Part model, mm, in its own coordinate system. A direction names the side the tool comes from. Give positions to 0.01 mm unless a question says otherwise; leave off trailing zeros. Write each loop counter-clockwise with the first axis right and the second up, starting at its lowest first coordinate (ties: lowest second). Pieces come first, ordered by that corner, then holes. Notation, with made-up numbers: M -36,-34.75 L 8,-34.75 A18 ccw 8,-11.75 Z; hole C -27.5,89.5 d10. An arc over 180 degrees is marked long. Write item = value, one per line. Start each with the question number.
from build123d import *

# Parameters (mm, degrees)
BOSS_EXTRUDE1_DEPTH = 127
CUT_EXTRUDE1_REACH  = 147.912
SKETCH2_R           = 6
SKETCH2_R_2         = 3.175
CUT_EXTRUDE2_REACH  = 147.912
SKETCH3_R           = 2.75
SKETCH3_W           = 29.8
SKETCH3_H           = 64.8
FILLET1_R           = 2


with BuildPart() as part:
    # Sketch1 → Boss-Extrude1 (new body)
    with BuildSketch(Plane(origin=(0, 0, 0), x_dir=(1, 0, 0), z_dir=(0, 1, 0))):
        Polygon((0, 50.8), (0, 0), (50.8, 0), (50.8, -3.175), (-3.175, -3.175), (-3.175, 50.8), align=None)
    extrude(amount=BOSS_EXTRUDE1_DEPTH)

    # Sketch2 → Cut-Extrude1 (cut, up to next)
    with BuildSketch(Plane(origin=(0, 0, 0), x_dir=(-1, 0, 0), z_dir=(0, 0, -1)), mode=Mode.PRIVATE) as cut_extrude1_sk1:
        with Locations((-25.4, 63.5)):
            Circle(SKETCH2_R)
    cut_extrude1_tool1 = extrude(cut_extrude1_sk1.sketch, amount=-CUT_EXTRUDE1_REACH, mode=Mode.PRIVATE) & part.part
    # Sketch2 → Cut-Extrude1 (cut, up to next)
    with BuildSketch(Plane(origin=(0, 0, 0), x_dir=(-1, 0, 0), z_dir=(0, 0, -1)), mode=Mode.PRIVATE) as cut_extrude1_sk2:
        with Locations((-25.4, 75.5)):
            Circle(SKETCH2_R_2)
    cut_extrude1_tool2 = extrude(cut_extrude1_sk2.sketch, amount=-CUT_EXTRUDE1_REACH, mode=Mode.PRIVATE) & part.part
    # Sketch2 → Cut-Extrude1 (cut, up to next)
    with BuildSketch(Plane(origin=(0, 0, 0), x_dir=(-1, 0, 0), z_dir=(0, 0, -1)), mode=Mode.PRIVATE) as cut_extrude1_sk3:
        with Locations((-13.4, 63.5)):
            Circle(SKETCH2_R_2)
    cut_extrude1_tool3 = extrude(cut_extrude1_sk3.sketch, amount=-CUT_EXTRUDE1_REACH, mode=Mode.PRIVATE) & part.part
    # Sketch2 → Cut-Extrude1 (cut, up to next)
    with BuildSketch(Plane(origin=(0, 0, 0), x_dir=(-1, 0, 0), z_dir=(0, 0, -1)), mode=Mode.PRIVATE) as cut_extrude1_sk4:
        with Locations((-25.4, 51.5)):
            Circle(SKETCH2_R_2)
    cut_extrude1_tool4 = extrude(cut_extrude1_sk4.sketch, amount=-CUT_EXTRUDE1_REACH, mode=Mode.PRIVATE) & part.part
    # Sketch2 → Cut-Extrude1 (cut, up to next)
    with BuildSketch(Plane(origin=(0, 0, 0), x_dir=(-1, 0, 0), z_dir=(0, 0, -1)), mode=Mode.PRIVATE) as cut_extrude1_sk5:
        with Locations((-37.4, 63.5)):
            Circle(SKETCH2_R_2)
    cut_extrude1_tool5 = extrude(cut_extrude1_sk5.sketch, amount=-CUT_EXTRUDE1_REACH, mode=Mode.PRIVATE) & part.part
    add(cut_extrude1_tool1.solids().sort_by_distance((25.4, 63.5, 0))[0], mode=Mode.SUBTRACT)
    add(cut_extrude1_tool2.solids().sort_by_distance((25.4, 75.5, 0))[0], mode=Mode.SUBTRACT)
    add(cut_extrude1_tool3.solids().sort_by_distance((13.4, 63.5, 0))[0], mode=Mode.SUBTRACT)
    add(cut_extrude1_tool4.solids().sort_by_distance((25.4, 51.5, 0))[0], mode=Mode.SUBTRACT)
    add(cut_extrude1_tool5.solids().sort_by_distance((37.4, 63.5, 0))[0], mode=Mode.SUBTRACT)

    # Sketch3 → Cut-Extrude2 (cut, up to next)
    with BuildSketch(Plane(origin=(0, 0, 0), x_dir=(0, 0, -1), z_dir=(1, 0, 0)), mode=Mode.PRIVATE) as cut_extrude2_sk1:
        with Locations((33.9, 100.9)):
            Circle(SKETCH3_R)
    cut_extrude2_tool1 = extrude(cut_extrude2_sk1.sketch, amount=-CUT_EXTRUDE2_REACH, mode=Mode.PRIVATE) & part.part
    # Sketch3 → Cut-Extrude2 (cut, up to next)
    with BuildSketch(Plane(origin=(0, 0, 0), x_dir=(0, 0, -1), z_dir=(1, 0, 0)), mode=Mode.PRIVATE) as cut_extrude2_sk2:
        with Locations((16.9, 100.9)):
            Circle(SKETCH3_R)
    cut_extrude2_tool2 = extrude(cut_extrude2_sk2.sketch, amount=-CUT_EXTRUDE2_REACH, mode=Mode.PRIVATE) & part.part
    # Sketch3 → Cut-Extrude2 (cut, up to next)
    with BuildSketch(Plane(origin=(0, 0, 0), x_dir=(0, 0, -1), z_dir=(1, 0, 0)), mode=Mode.PRIVATE) as cut_extrude2_sk3:
        with Locations((16.9, 26.1)):
            Circle(SKETCH3_R)
    cut_extrude2_tool3 = extrude(cut_extrude2_sk3.sketch, amount=-CUT_EXTRUDE2_REACH, mode=Mode.PRIVATE) & part.part
    # Sketch3 → Cut-Extrude2 (cut, up to next)
    with BuildSketch(Plane(origin=(0, 0, 0), x_dir=(0, 0, -1), z_dir=(1, 0, 0)), mode=Mode.PRIVATE) as cut_extrude2_sk4:
        with Locations((33.9, 26.1)):
            Circle(SKETCH3_R)
    cut_extrude2_tool4 = extrude(cut_extrude2_sk4.sketch, amount=-CUT_EXTRUDE2_REACH, mode=Mode.PRIVATE) & part.part
    # Sketch3 → Cut-Extrude2 (cut, up to next)
    with BuildSketch(Plane(origin=(0, 0, 0), x_dir=(0, 0, -1), z_dir=(1, 0, 0)), mode=Mode.PRIVATE) as cut_extrude2_sk5:
        with Locations((25.4, 63.5)):
            Rectangle(SKETCH3_W, SKETCH3_H)
    cut_extrude2_tool5 = extrude(cut_extrude2_sk5.sketch, amount=-CUT_EXTRUDE2_REACH, mode=Mode.PRIVATE) & part.part
    add(cut_extrude2_tool1.solids().sort_by_distance((0, 100.9, -33.9))[0], mode=Mode.SUBTRACT)
    add(cut_extrude2_tool2.solids().sort_by_distance((0, 100.9, -16.9))[0], mode=Mode.SUBTRACT)
    add(cut_extrude2_tool3.solids().sort_by_distance((0, 26.1, -16.9))[0], mode=Mode.SUBTRACT)
    add(cut_extrude2_tool4.solids().sort_by_distance((0, 26.1, -33.9))[0], mode=Mode.SUBTRACT)
    add(cut_extrude2_tool5.solids().sort_by_distance((0, 63.5, -25.4))[0], mode=Mode.SUBTRACT)

    # Fillet1
    fillet1_edges = [part.edges().sort_by_distance(p)[0] for p in [
        (0, 63.5, 0),
    ]]
    fillet(fillet1_edges, radius=FILLET1_R)


solid = part.part
Q1. Slice it at A-A (z = -33.9). Give the cut face in (x, y) (3 decimals).
Q2. Probe line 1 along Z through (x, y) = (-1, 26) (3 decimals); line 2 along Y through (x, z) = (25.4, 2.2) (3 decimals); line 3 along Y through (x, z) = (25, 2). List the from-to ranges inside material, lowest first.
Q3. Drop flat-ended pins along their axis: P1, Ø3.5, axis at y = 26.1, z = -16.9, coming from the -X side (3 decimals); P2, Ø10, axis at x = 25.4, y = 75.5, coming from the -Z side; P3, Ø8, axis at y = 77, z = -6, coming from the +X side; P4, Ø6.5, axis at y = 26.1, z = -33.9, coming from the -X side (3 decimals). Give the stop position or say it passes through.
Q4. Slice it at B-B (y = 82.5). Give the cut face in (x, z) (3 decimals), and give its area (3 significant figures).
Q5. Slice it at D-D (y = 26.1). Give the cut face in (x, z) (3 decimals), and give its area (3 significant figures).
Q6. Two-plate mould, pull along Z, no slides. Class faces 3 (the face through (23.9, 48.7, 1.6)), 4 (the face through (31.5, 62.6, 0)), 5 (the face through (-1.565, 23.415, -33.304)): +Z half, -Z half, draft (parallel to the pull), parting line (faces both ways), or undercut.
Q7. Tool access for faces 1 (the face through (-2, 95.9, -25)), 2 (the face through (15.74, 65.646, 1.565)): list every direction of +Z, -Z, +X, -X, +Y, -Y with a clear straight run to the whole face (end or side of a thin tool).
Q8. Slice it at C-C (x = 13.4). Give the cut face in (y, z) (3 decimals), and give its area (3 significant figures).
Working result:
q1.outline = M -3.175,0 L 0,0 L 0,23.35 L -3.175,23.35 Z; M -3.175,28.85 L 0,28.85 L 0,31.1 L -3.175,31.1 Z; M -3.175,95.9 L 0,95.9 L 0,98.15 L -3.175,98.15 Z; M -3.175,103.65 L 0,103.65 L 0,127 L -3.175,127 Z
q2.line_1 = -50.8 to -36.648, -31.152 to -19.648, -14.152 to 3.175
q2.line_2 = 0 to 48.325, 54.675 to 57.5, 69.5 to 72.325, 78.675 to 127
q2.line_3 = 0 to 48.35, 54.65 to 57.51, 69.49 to 72.35, 78.65 to 127
q3.P1 = through
q3.P2 = 0
q3.P3 = 0
q3.P4 = -3.175
q4.outline = M -3.175,-50.8 L 0,-50.8 L 0,-40.3 L -3.175,-40.3 Z; M -3.175,-10.5 L 0,-10.5 L 0,-2 A2 cw 2,0 L 50.8,0 L 50.8,3.175 L -3.175,3.175 Z
q4.area = 239 mm2
q5.outline = M -3.175,-50.8 L 0,-50.8 L 0,-36.65 L -3.175,-36.65 Z; M -3.175,-31.15 L 0,-31.15 L 0,-19.65 L -3.175,-19.65 Z; M -3.175,-14.15 L 0,-14.15 L 0,-2 A2 cw 2,0 L 50.8,0 L 50.8,3.175 L -3.175,3.175 Z
q5.area = 299 mm2
q6.face_3 = draft
q6.face_4 = -Z half
q6.face_5 = undercut
q7.face_1 = +X, -X
q7.face_2 = +Z, -Z
q8.outline = M 0,0 L 60.325,0 L 60.325,3.175 L 0,3.175 Z; M 66.675,0 L 127,0 L 127,3.175 L 66.675,3.175 Z
q8.area = 383 mm2
